```python
from build123d import *

# Parameters (mm, degrees)
SKETCH2_R                = 2.5
SKETCH2_R_2              = 1.5
BOSS_EXTRUDE1_DEPTH      = 1.95
SKETCH3_W                = 5
SKETCH3_H                = 10
BOSS_EXTRUDE2_DEPTH      = 1
BOSS_EXTRUDE2_DEPTH_BACK = 1
SKETCH5_R                = 2.5
SKETCH5_R_2              = 1.50060411
BOSS_EXTRUDE3_DEPTH      = 0.975
BOSS_EXTRUDE3_DEPTH_BACK = 0.975
SKETCH6_W                = 1.95
SKETCH6_H                = 2
BOSS_EXTRUDE4_DEPTH      = 0.208712
SKETCH7_R                = 1
CUT_EXTRUDE1_DEPTH       = 10


with BuildPart() as part:
    # Sketch2 → Boss-Extrude1 (new body)
    with BuildSketch(Plane.XY):
        Circle(SKETCH2_R)
        Circle(SKETCH2_R_2, mode=Mode.SUBTRACT)
    extrude(amount=BOSS_EXTRUDE1_DEPTH)



with BuildPart() as body_2:
    # Sketch3 → Boss-Extrude2 (new body, two sides)
    with BuildSketch(Plane(origin=(0, 0, 0), x_dir=(1, 0, 0), z_dir=(0, 1, 0))) as boss_extrude2_sk:
        with Locations((-5, -2.975)):
            Rectangle(SKETCH3_W, SKETCH3_H)
    extrude(amount=BOSS_EXTRUDE2_DEPTH)
    extrude(boss_extrude2_sk.sketch, amount=-BOSS_EXTRUDE2_DEPTH_BACK)


with BuildPart() as body_3:
    # Sketch5 → Boss-Extrude3 (new body, two sides)
    with BuildSketch(Plane(origin=(0, 0, 4.975), x_dir=(0, -1, 0), z_dir=(0, 0, 1))) as boss_extrude3_sk:
        Circle(SKETCH5_R)
        Circle(SKETCH5_R_2, mode=Mode.SUBTRACT)
    extrude(amount=BOSS_EXTRUDE3_DEPTH)
    extrude(boss_extrude3_sk.sketch, amount=-BOSS_EXTRUDE3_DEPTH_BACK)


with BuildPart() as part_1:
    add(part.part)

    add(body_2.part)  # Boss-Extrude4 merges body 2

    add(body_3.part)  # Boss-Extrude4 merges body 3
    # Sketch6 → Boss-Extrude4 (add)
    with BuildSketch(Plane(origin=(-2.5, 0, 0), x_dir=(0, 0, -1), z_dir=(1, 0, 0))):
        with Locations((-4.975, 0)):
            Rectangle(SKETCH6_W, SKETCH6_H)
        with Locations((-0.975, 0)):
            Rectangle(SKETCH6_W, SKETCH6_H)
    extrude(amount=BOSS_EXTRUDE4_DEPTH)

    # Sketch7 → Cut-Extrude1 (cut)
    with BuildSketch(Plane(origin=(0, 1, 0), x_dir=(1, 0, 0), z_dir=(0, 1, 0))):
        with Locations((-5, -5.475)):
            Circle(SKETCH7_R)
        with Locations((-5, -0.475)):
            Circle(SKETCH7_R)
    extrude(amount=-CUT_EXTRUDE1_DEPTH, mode=Mode.SUBTRACT)


solid = part_1.part
```
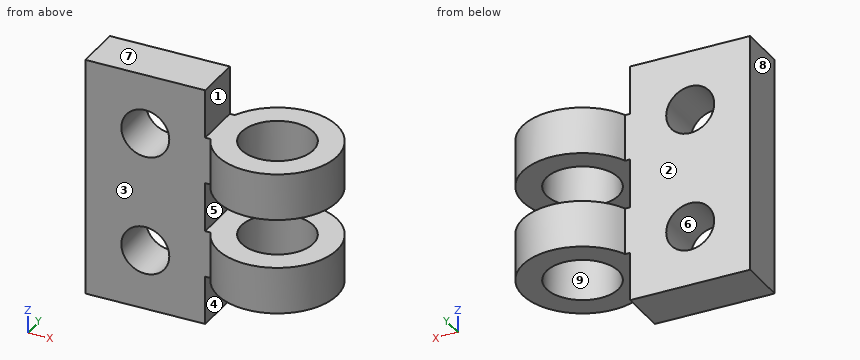
The listing builds one solid part. Answer for the finished solid, in the listing's coordinates (mm). Face numbers are marked on the shaded views. A direction names the side the tool comes from. Round coordinates to 2 decimals unless told otherwise and drop trailing zeros. Order: outer loops, then holes, each group sorted by start corner. A loop starts at its lowest first (then second) coordinate and runs counter-clockwise, first axis right, second up. Notation, with made-up numbers: (-34.5, 66) - (10.5, 66) arc R30 cw to (10.5, 94) - close; hole circle Ø2 at (12.25, 28). An arc over 180 degrees is marked (long way). Put each result on its own line as item: value. Start each with the question number.
(1) Find section A-A (y = 0). Give the vertices of the cut face in (x, z) (3 decimals), plus the area to 3 significant figures.
(2) Given P1, Ø2.5, axis at x = -5, z = 0.475, coming from the -Y side; P2, Ø2.5, axis at x = -6, z = 1, coming from the +Y side; P3, Ø1, axis at x = -1, y = -0.5, coming from the -Z side, each flat-ended and moving along its own axis, determine where each tip first touches the part or whether it passes through.
(3) Find section B-B (x = 0). Give the vertices of the cut face in (y, z), plus the area to 3 significant figures.
(4) For the marked faces 1, 2, 3, 4 and 5, determine the directions among +Z, -Z, +X, -X, +Y, -Y from which every point of the face is accessible in a straight line to the end or side of a thin tool.
(5) Find section D-D (y = 2). Give the vertices of the cut face in (x, z).
(6) Determine the mould class of the marked faces 6, 7, 8 and 9 for opening direction X: released by +X, released by -X, zero draft, split by the parting line, or undercut.
(7) Find section C-C (x = -5). Give the vertices of the cut face in (y, z) (3 decimals), plus the area to 3 significant figures.
(8) Straight lines are drawn through the part: probe 1 along Z at (x, y) = (-5, -0.25) (3 decimals); probe 2 along Z at (x, y) = (-0.25, 1.7); probe 3 along X at (y, z) = (0, 5.5). For each, find the intervals that lie inside material, in ascending order. Write a range as from..to.
Reply:
1. outline: (-7.5, -2.025) - (-2.5, -2.025) - (-2.5, 0) - (-1.5, 0) - (-1.5, 1.95) - (-2.5, 1.95) - (-2.5, 4) - (-1.501, 4) - (-1.501, 5.95) - (-2.5, 5.95) - (-2.5, 7.975) - (-7.5, 7.975) - close; (1.5, 0) - (2.5, 0) - (2.5, 1.95) - (1.5, 1.95) - close; (1.501, 4) - (2.5, 4) - (2.5, 5.95) - (1.501, 5.95) - close; hole circle Ø2 at (-5, 0.475); hole circle Ø2 at (-5, 5.475)
1. area: 51.5 mm^2
2. P1: y = -1
2. P2: y = 1
2. P3: z = 0
3. outline: (-2.5, 0) - (-1.5, 0) - (-1.5, 1.95) - (-2.5, 1.95) - close; (-2.5, 4) - (-1.5, 4) - (-1.5, 5.95) - (-2.5, 5.95) - close; (1.5, 0) - (2.5, 0) - (2.5, 1.95) - (1.5, 1.95) - close; (1.5, 4) - (2.5, 4) - (2.5, 5.95) - (1.5, 5.95) - close
3. area: 7.80 mm^2
4. face 1: +Z, +X, +Y, -Y
4. face 2: +Z, -Z, -X, +Y
4. face 3: +Z, -Z, -X, -Y
4. face 4: -Z, +X, +Y, -Y
4. face 5: +X, +Y, -Y
5. outline: (-1.5, 0) - (1.5, 0) - (1.5, 1.95) - (-1.5, 1.95) - close; (-1.5, 4) - (1.5, 4) - (1.5, 5.95) - (-1.5, 5.95) - close
6. face 6: undercut
6. face 7: zero draft
6. face 8: released by -X
6. face 9: undercut
7. outline: (-1, -2.025) - (1, -2.025) - (1, -0.525) - (-1, -0.525) - close; (-1, 1.475) - (1, 1.475) - (1, 4.475) - (-1, 4.475) - close; (-1, 6.475) - (1, 6.475) - (1, 7.975) - (-1, 7.975) - close
7. area: 12.0 mm^2
8. probe 1: -2.025..-0.525, 1.475..4.475, 6.475..7.975
8. probe 2: 0..1.95, 4..5.95
8. probe 3: -7.5..-6, -4..-1.5, 1.5..2.5
